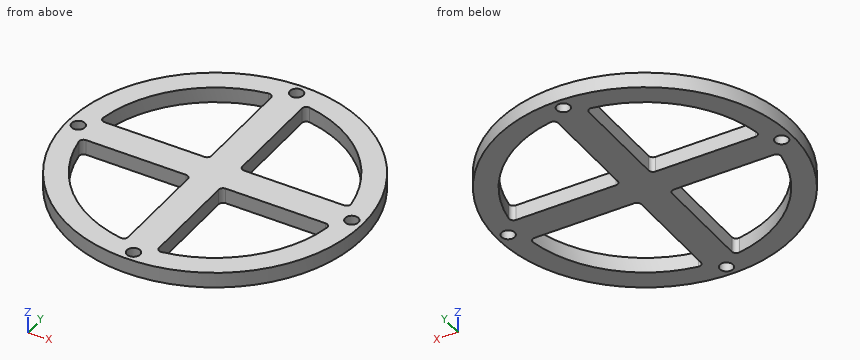
from build123d import *

# Parameters (mm, degrees)
SCHIZZO2_R                   = 67
ESTRUSIONE_ESTRUSIONE1_DEPTH = 7
SCHIZZO3_R                   = 3
TAGLIO_ESTRUSIONE2_DEPTH     = 7
RIPETIZIONECIRCOLARE1_COUNT  = 4


with BuildPart() as part:
    # Schizzo2 → Estrusione-Estrusione1 (new body)
    with BuildSketch(Plane.XY):
        Circle(SCHIZZO2_R)
        with BuildLine():
            Line((7, 9), (7, 54.258639865))
            ThreePointArc((7, 54.258639865), (7.706660419, 55.784180008), (9.327272727, 56.231681315))
            ThreePointArc((9.327272727, 56.231681315), (40.305086528, 40.305086528), (56.231681315, 9.327272727))
            ThreePointArc((56.231681315, 9.327272727), (55.784180008, 7.706660419), (54.258639865, 7))
            Line((54.258639865, 7), (9, 7))
            ThreePointArc((9, 7), (7.585786438, 7.585786438), (7, 9))
        make_face(mode=Mode.SUBTRACT)
        with BuildLine():
            Line((-9, 7), (-54.258639865, 7))
            ThreePointArc((-54.258639865, 7), (-55.784180008, 7.706660419), (-56.231681315, 9.327272727))
            ThreePointArc((-56.231681315, 9.327272727), (-40.305086528, 40.305086528), (-9.327272727, 56.231681315))
            ThreePointArc((-9.327272727, 56.231681315), (-7.706660419, 55.784180008), (-7, 54.258639865))
            Line((-7, 54.258639865), (-7, 9))
            ThreePointArc((-7, 9), (-7.585786438, 7.585786438), (-9, 7))
        make_face(mode=Mode.SUBTRACT)
        with BuildLine():
            Line((-9, -7), (-54.258639865, -7))
            ThreePointArc((-54.258639865, -7), (-55.784180008, -7.706660419), (-56.231681315, -9.327272727))
            ThreePointArc((-56.231681315, -9.327272727), (-40.305086528, -40.305086528), (-9.327272727, -56.231681315))
            ThreePointArc((-9.327272727, -56.231681315), (-7.706660419, -55.784180008), (-7, -54.258639865))
            Line((-7, -54.258639865), (-7, -9))
            ThreePointArc((-7, -9), (-7.585786438, -7.585786438), (-9, -7))
        make_face(mode=Mode.SUBTRACT)
        with BuildLine():
            Line((7, -54.258639865), (7, -9))
            ThreePointArc((7, -9), (7.585786438, -7.585786438), (9, -7))
            Line((9, -7), (54.258639865, -7))
            ThreePointArc((54.258639865, -7), (55.784180008, -7.706660419), (56.231681315, -9.327272727))
            ThreePointArc((56.231681315, -9.327272727), (40.305086528, -40.305086528), (9.327272727, -56.231681315))
            ThreePointArc((9.327272727, -56.231681315), (7.706660419, -55.784180008), (7, -54.258639865))
        make_face(mode=Mode.SUBTRACT)
    extrude(amount=ESTRUSIONE_ESTRUSIONE1_DEPTH)

    # Schizzo3 → Taglio-Estrusione2 (cut)
    with BuildSketch(Plane.XY):
        with Locations((0, 62)):
            Circle(SCHIZZO3_R)
    taglio_estrusione2 = extrude(amount=TAGLIO_ESTRUSIONE2_DEPTH, mode=Mode.SUBTRACT)

    # RipetizioneCircolare1: Taglio-Estrusione2 ×4 about axis
    ripetizionecircolare1_axis = Axis((0, 0, 0), (0, 0, 1))
    for i in range(1, RIPETIZIONECIRCOLARE1_COUNT):
        add(taglio_estrusione2.rotate(ripetizionecircolare1_axis, i * 360 / RIPETIZIONECIRCOLARE1_COUNT), mode=Mode.SUBTRACT)


solid = part.part
The listing builds one solid part. Answer for the finished solid, in the listing's coordinates (mm). Give positions to 0.01 mm unless a question says otherwise; leave off trailing zeros. Write each loop counter-clockwise with the first axis right and the second up, starting at its lowest first coordinate (ties: lowest second). Pieces come first, ordered by that corner, then holes.
Item 1: Section A-A, the plane y = 0 is taken. Write down the section's boundary in (x, z).
Item 2: Find the intervals of material crossed by line 1 along Y through (x, z) = (0, 3.25); line 2 along X through (y, z) = (-43.5, 2.75); line 3 along Y through (x, z) = (-20.5, 3), in increasing order.
Item 3: Section C-C, the plane z = 4.5 is taken. Count the separate pieces of the cut face and the enclosed holes in it, plus the area to 3 significant figures.
Item 4: Flat-ended cylindrical pins translate along their axes: P1, Ø2, axis at y = -35, z = 2, coming from the -X side; P2, Ø3.5, axis at y = -27, z = 3.5, coming from the +X side; P3, Ø9.5, axis at x = 62, y = 0, coming from the +Z side; P4, Ø12, axis at x = 37, y = -31, coming from the -Z side. Find the tip coordinate at first contact, or state that the pin passes through.
Item 5: Section D-D, the plane y = 62 is taken. Write down the section's boundary in (x, z), plus the area to 3 significant figures.
Completed:
1. outline: (-67, 0) - (-65, 0) - (-65, 7) - (-67, 7) - close; (-59, 0) - (59, 0) - (59, 7) - (-59, 7) - close; (65, 0) - (67, 0) - (67, 7) - (65, 7) - close
2. line 1: y = -67 to -65, -59 to 59, 65 to 67
2. line 2: x = -50.96 to -36.83, -7 to 7, 36.83 to 50.96
2. line 3: y = -63.79 to -53.19, -7 to 7, 53.19 to 63.79
3. separate pieces: 1
3. enclosed holes: 8
3. area: 6,780 mm2
4. P1: stops at x = -57.73
4. P2: stops at x = 62.06
4. P3: stops at z = 7
4. P4: passes through
5. outline: (-25.4, 0) - (-3, 0) - (-3, 7) - (-25.4, 7) - close; (3, 0) - (25.4, 0) - (25.4, 7) - (3, 7) - close
5. area: 314 mm2
